```python
from build123d import *

# Parameters (mm, degrees)
SKETCH2_W               = 3
SKETCH2_H               = 3
CUT_EXTRUDE1_DEPTH      = 13
CUT_EXTRUDE1_DEPTH_BACK = 13
CHAMFER1_SIZE           = 1


with BuildPart() as part:
    # Sketch1 → Revolve1 (revolve)
    with BuildSketch(Plane.XY):
        Polygon((0, 40), (12, 40), (12, 31), (8, 31), (8, 11), (5.25, 11), (5.25, 9), (6, 7.700961894), (6, 0), (0, 0), align=None)
    revolve(axis=Axis((0, 0, 0), (0, 1, 0)))

    # Sketch2 → Cut-Extrude1 (cut, two sides)
    with BuildSketch(Plane.XY) as cut_extrude1_sk:
        with Locations((0, 38.5)):
            Rectangle(SKETCH2_W, SKETCH2_H)
    extrude(amount=CUT_EXTRUDE1_DEPTH, mode=Mode.SUBTRACT)
    extrude(cut_extrude1_sk.sketch, amount=-CUT_EXTRUDE1_DEPTH_BACK, mode=Mode.SUBTRACT)

    # Chamfer1
    chamfer1_edges = [part.edges().sort_by_distance(p)[0] for p in [
        (9, 40, -7.937253933),
        (-12, 40, 0),
    ]]
    chamfer(chamfer1_edges, length=CHAMFER1_SIZE)


solid = part.part
```
For this review, take the finished solid that the model builds, in its own axes (mm). A direction names the side the tool comes from. Give positions to 0.01 mm unless a question says otherwise; leave off trailing zeros. Loops run counter-clockwise (first coordinate to the right, second up) from the corner with the lowest first, then second, coordinate; pieces in that order, holes last. Notation, with made-up numbers: M 87.25,-25 L 125.25,-25 A13 cw 125.25,-5 Z; hole C -11.75,14 d8. An arc over 180 degrees is marked long. One line per item, written item: value. Start each with the question number.
Q1. For L1, parallel to Y at x = -9.75, z = -4; L2, parallel to Z at x = 0, y = 22; L3, parallel to Y at x = -0.75, z = -0.5, list the stretches that pass through material, from the lowest coordinate up.
Q2. Add section D-D (y = 5). Give the boundary of the cut face in (x, z), and give its area (3 significant figures).
Q3. Clearance check with flat-ended pins moving along their axes: pin 1 Ø2.5 at (x, z) = (0.5, 3) entering from +Y; pin 2 Ø4 at (y, z) = (16.5, 3.5) entering from +X; pin 3 Ø1.5 at (y, z) = (33.5, 1) entering from -X; pin 4 Ø1 at (x, y) = (-7, 26) entering from +Z. State where each tip first meets the part, or that it passes through.
Q4. Add section A-A (x = 0). Give the boundary of the cut face in (y, z).
Q5. Machinability: for faces 5 (the face through (0, 37, 0)), 6 (the face through (-1.73, 20.86, 7.81)), 7 (the face through (-5, 40, 0)), which of the approach directions +Z, -Z, +X, -X, +Y, -Y give a long, thin tool a straight path to every point of the face, cutting with its end or side? Answer none if there is none.
Q6. Add section C-C (y = 29.5). Give the boundary of the cut face in (x, z), and give its area (3 significant figures).
Q7. Draft analysis for pull direction Y (two halves, no side actions). For faces 1 (the face through (11.2, 39.8, 0.2)), 2 (the face through (5, 10, -1.6)), 3 (the face through (-1.5, 38, 0)), 4 (the face through (5.2, 11, 1.7)), state which applies: released by +Y, released by -Y, zero draft, split by the parting line, or undercut.
Q8. Add section B-B (z = 0). Give the boundary of the cut face in (x, y), and give its area (3 significant figures).
Reply:
1. L1: 31 to 40
1. L2: -8 to 8
1. L3: 0 to 37
2. outline: C 0,0 d12
2. area: 113 mm²
3. pin 1: y = 40
3. pin 2: x = 7.86
3. pin 3: x = -12
3. pin 4: z = 4.66
4. outline: M 0,-6 L 7.7,-6 L 9,-5.25 L 11,-5.25 L 11,-8 L 31,-8 L 31,-12 L 37,-12 L 37,12 L 31,12 L 31,8 L 11,8 L 11,5.25 L 9,5.25 L 7.7,6 L 0,6 Z
5. face 5: +Z, -Z, +Y
5. face 6: -Y
5. face 7: +Z, -Z, +X, -X, +Y
6. outline: C 0,0 d16
6. area: 201 mm²
7. face 1: released by +Y
7. face 2: undercut
7. face 3: zero draft
7. face 4: undercut
8. outline: M -12,31 L -8,31 L -8,11 L -5.25,11 L -5.25,9 L -6,7.7 L -6,0 L 6,0 L 6,7.7 L 5.25,9 L 5.25,11 L 8,11 L 8,31 L 12,31 L 12,39 L 11,40 L 1.5,40 L 1.5,37 L -1.5,37 L -1.5,40 L -11,40 L -12,39 Z
8. area: 654 mm²
